Geometry check sheet. Reference: the model listing, model coordinates, mm. A direction names the side the tool comes from. Coordinates: 2 decimals unless noted, no trailing zeros. Loops run counter-clockwise (first coordinate to the right, second up) from the corner with the lowest first, then second, coordinate; pieces in that order, holes last.
from build123d import *

# Parameters (mm, degrees)
SKETCH1_W           = 10
SKETCH1_H           = 5
BOSS_EXTRUDE1_DEPTH = 2.5


with BuildPart() as part:
    # Sketch1 → Boss-Extrude1 (new, symmetric)
    with BuildSketch(Plane.YZ):
        Polygon((75, 0), (65, 0), (0, 0), (0, -5), (162, -5), (162, 0), (135, 0), (125, 0), align=None)
        with Locations((70, 2.5)):
            Rectangle(SKETCH1_W, SKETCH1_H)
        with Locations((130, 2.5)):
            Rectangle(SKETCH1_W, SKETCH1_H)
    boss_extrude1 = extrude(amount=BOSS_EXTRUDE1_DEPTH, both=True)

    # Mirror1: Boss-Extrude1 across plane
    add(boss_extrude1.mirror(Plane.ZX))


solid = part.part
1) Material ranges on probe 1 along Y at (x, z) = (0.95, 2.25); probe 2 along Z at (x, y) = (-1.85, 46), recorded low to high.
Data:
probe 1: y = -135 to -125, -75 to -65, 65 to 75, 125 to 135
probe 2: z = -5 to 0
2) Section check A-A on z = 2.25. Record the cut outline in (x, y), and give its area (3 significant figures).
Data:
outline: (-2.5, -135) - (2.5, -135) - (2.5, -125) - (-2.5, -125) - close; (-2.5, -75) - (2.5, -75) - (2.5, -65) - (-2.5, -65) - close; (-2.5, 65) - (2.5, 65) - (2.5, 75) - (-2.5, 75) - close; (-2.5, 125) - (2.5, 125) - (2.5, 135) - (-2.5, 135) - close
area: 200 mm2
3) Depth check by flat-ended pin: pin 1 (3 mm diameter, centred on x = 0.5, z = 4, fed in from -Y); pin 2 (1.5 mm diameter, centred on x = -1, y = 0.5, fed in from +Z); pin 3 (1.5 mm diameter, centred on x = 0.5, z = 2.5, fed in from +Y). Enter the tip coordinate at first touch or a pass-through.
Data:
pin 1: stops at y = -135
pin 2: stops at z = 0
pin 3: stops at y = 135
4) Section check C-C on y = -42. Record the cut outline in (x, z).
Data:
outline: (-2.5, -5) - (2.5, -5) - (2.5, 0) - (-2.5, 0) - close
5) Mould release check, pull along Y, two halves, no side actions. Record for faces 1 (the flat face through (0, -135, 2)), 2 (the flat face through (0, 162, -3)), 3 (the flat face through (0, 100, 0)): +Y half, -Y half, draft (parallel to the pull), parting line (faces both ways), or undercut.
Data:
face 1: -Y half
face 2: +Y half
face 3: undercut
6) Section check B-B on x = 0.85. Record the cut outline in (y, z).
Data:
outline: (-162, -5) - (162, -5) - (162, 0) - (135, 0) - (135, 5) - (125, 5) - (125, 0) - (75, 0) - (75, 5) - (65, 5) - (65, 0) - (-65, 0) - (-65, 5) - (-75, 5) - (-75, 0) - (-125, 0) - (-125, 5) - (-135, 5) - (-135, 0) - (-162, 0) - close
7) Access from +Z, -Z, +X, -X, +Y, -Y to the whole of each face (thin tool, end or side, straight path). Record for faces 4 (the flat face through (0, 70, 5)), 5 (the flat face through (0, -75, 2)), 6 (the flat face through (0, 135, 2)), 7 (the flat face through (0, -149, 0)).
Data:
face 4: +Z, +X, -X, +Y, -Y
face 5: +Z, +X, -X
face 6: +Z, +X, -X, +Y
face 7: +Z, +X, -X, -Y
